The model under review builds one solid part; all positions refer to its coordinate system, in mm. Coordinates: 2 decimals unless noted, no trailing zeros. Loops run counter-clockwise (first coordinate to the right, second up) from the corner with the lowest first, then second, coordinate; pieces in that order, holes last. Notation, with made-up numbers: (-31, 9.25) - (-19, 9.25) arc R28 ccw to (-19, 40.25) - close; hole circle Ø8 at (63.5, -8.5). An arc over 180 degrees is marked (long way). One line per item, written item: value. Start each with the question number.
1. We need section B-B, the plane x = -27.5. Give the boundary of the cut face in (y, z), then the cut area to 3 significant figures.
2. We need section A-A, the plane y = -19.5. Give the boundary of the cut face in (x, z).
3. We need section D-D, the plane x = 9.5. Give the boundary of the cut face in (y, z), then the cut area to 3 significant figures.
4. Mouldability with a two-part tool opening along X and no side actions: class faces 1 (the face through (28.23, -16.16, 1.88)), 2 (the face through (-11, -18, 3.81)), 3 (the face through (40.314, -18, 2)), 4 (the face through (9.248, -15.117, 1.878)) as +X half, -X half, draft (parallel to the pull), parting line (faces both ways), or undercut.
5. Insertion check: P1, Ø1, axis at x = -49.5, y = -16.5, coming from the -Z side. The pin has a flat end and moves straight along its axis. Give the tip position at first contact, or say it passes through.
6. To check wall thickness, follow line 1 (X direction, y = -18.5, z = 0.9); line 2 (X direction, y = -19.5, z = 1.7); line 3 (Y direction, x = 7, z = 0.8). State the ranges of each line that lie inside material, in increasing order.
7. We need section C-C, the plane z = 0.95. Give the boundary of the cut face in (x, y), then the cut area to 3 significant figures.
from build123d import *

# Parameters (mm, degrees)
SKETCH1_W           = 100.584
SKETCH1_H           = 12.7
SKETCH1_R           = 3.302
BOSS_EXTRUDE2_DEPTH = 3.81
CUT_EXTRUDE1_REACH  = 5.81
SKETCH2_R           = 3.302


with BuildPart() as part:
    # Sketch1 → Boss-Extrude2 (new body)
    with BuildSketch(Plane.XY):
        with Locations((-9.978006062, -18.390640797)):
            Rectangle(SKETCH1_W, SKETCH1_H)
        with Locations((30.661993938, -18.390640797)):
            Circle(SKETCH1_R, mode=Mode.SUBTRACT)
        with Locations((-50.618006062, -18.390640797)):
            Circle(SKETCH1_R, mode=Mode.SUBTRACT)
    extrude(amount=BOSS_EXTRUDE2_DEPTH)

    # Sketch2 → Cut-Extrude1 (cut, up to next)
    with BuildSketch(Plane(origin=(0, 0, 0), x_dir=(-1, 0, 0), z_dir=(0, 0, -1)), mode=Mode.PRIVATE) as cut_extrude1_sk1:
        with Locations((28.774006062, -18.390640797)):
            Circle(SKETCH2_R)
    cut_extrude1_tool1 = extrude(cut_extrude1_sk1.sketch, amount=-CUT_EXTRUDE1_REACH, mode=Mode.PRIVATE) & part.part
    add(cut_extrude1_tool1.solids().sort_by_distance((-28.774006, -18.390641, 0))[0], mode=Mode.SUBTRACT)
    # Sketch2 → Cut-Extrude1 (cut, up to next)
    with BuildSketch(Plane(origin=(0, 0, 0), x_dir=(-1, 0, 0), z_dir=(0, 0, -1)), mode=Mode.PRIVATE) as cut_extrude1_sk2:
        with Locations((-8.817993938, -18.390640797)):
            Circle(SKETCH2_R)
    cut_extrude1_tool2 = extrude(cut_extrude1_sk2.sketch, amount=-CUT_EXTRUDE1_REACH, mode=Mode.PRIVATE) & part.part
    add(cut_extrude1_tool2.solids().sort_by_distance((8.817994, -18.390641, 0))[0], mode=Mode.SUBTRACT)


solid = part.part
Findings below:
1. outline: (-24.74, 0) - (-21.44, 0) - (-21.44, 3.81) - (-24.74, 3.81) - close; (-15.34, 0) - (-12.04, 0) - (-12.04, 3.81) - (-15.34, 3.81) - close
1. area: 25.2 mm2
2. outline: (-60.27, 0) - (-53.73, 0) - (-53.73, 3.81) - (-60.27, 3.81) - close; (-47.51, 0) - (-31.88, 0) - (-31.88, 3.81) - (-47.51, 3.81) - close; (-25.66, 0) - (5.71, 0) - (5.71, 3.81) - (-25.66, 3.81) - close; (11.93, 0) - (27.55, 0) - (27.55, 3.81) - (11.93, 3.81) - close; (33.77, 0) - (40.31, 0) - (40.31, 3.81) - (33.77, 3.81) - close
3. outline: (-24.74, 0) - (-21.62, 0) - (-21.62, 3.81) - (-24.74, 3.81) - close; (-15.16, 0) - (-12.04, 0) - (-12.04, 3.81) - (-15.16, 3.81) - close
3. area: 23.8 mm2
4. face 1: undercut
4. face 2: draft
4. face 3: +X half
4. face 4: undercut
5. P1: through
6. line 1: -60.27 to -53.92, -47.32 to -32.07, -25.47 to 5.52, 12.12 to 27.36, 33.96 to 40.31
6. line 2: -60.27 to -53.73, -47.51 to -31.88, -25.66 to 5.71, 11.93 to 27.55, 33.77 to 40.31
6. line 3: -24.74 to -21.15, -15.63 to -12.04
7. outline: (-60.27, -24.74) - (40.31, -24.74) - (40.31, -12.04) - (-60.27, -12.04) - close; hole circle Ø6.6 at (-50.62, -18.39); hole circle Ø6.6 at (-28.77, -18.39); hole circle Ø6.6 at (8.82, -18.39); hole circle Ø6.6 at (30.66, -18.39)
7. area: 1,140 mm2
